Source: three-view drawing plus pictorial views. Frame: mm from the lowest corner of the part. A direction names the side the tool comes from. Give positions to 0.01 mm unless a question says otherwise; leave off trailing zeros. Loops run counter-clockwise (first coordinate to the right, second up) from the corner with the lowest first, then second, coordinate; pieces in that order, holes last. Notation, with made-up numbers: (68, -10.5) - (90, -10.5) arc R19 cw to (90, -1.5) - close; hole circle Ø7 at (-26, -5). An arc over 180 degrees is marked (long way). One line per item, written item: value.
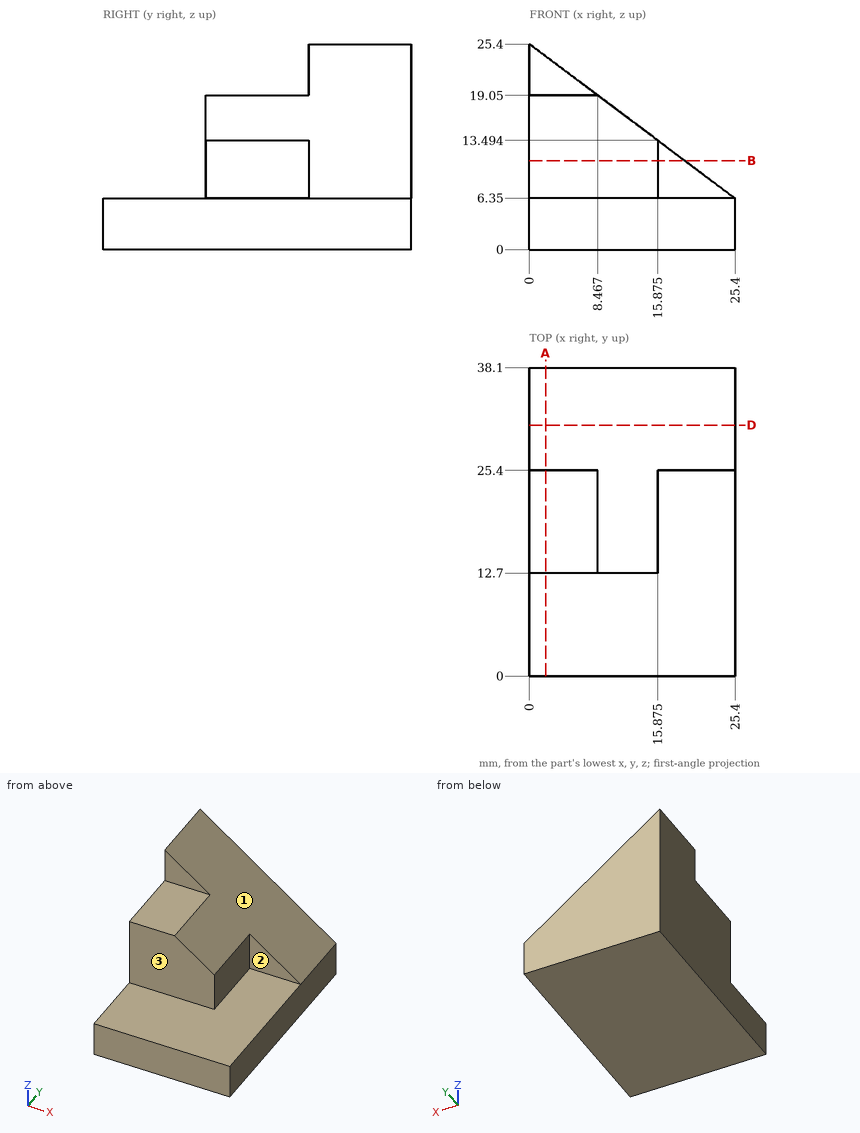
Item 1: Material intervals for L1, parallel to Z at x = 4.25, y = 6; L2, parallel to Z at x = 7.75, y = 14; L3, parallel to Y at x = 2.5, z = 10, sorted ascending.
Verdict:
L1: z = 0 to 6.35
L2: z = 0 to 19.05
L3: y = 12.7 to 38.1
Item 2: Section A-A, the plane x = 2. Output: boundary loops of the cut face in (y, z), and give its area (3 significant figures).
Verdict:
outline: (0, 0) - (38.1, 0) - (38.1, 23.9) - (25.4, 23.9) - (25.4, 19.05) - (12.7, 19.05) - (12.7, 6.35) - (0, 6.35) - close
area: 626 mm^2
Item 3: Section D-D, the plane y = 31. Output: boundary loops of the cut face in (x, z), and give its area (3 significant figures).
Verdict:
outline: (0, 0) - (25.4, 0) - (25.4, 6.35) - (0, 25.4) - close
area: 403 mm^2
Item 4: Access query for the marked faces 1, 2 and 3. Directions: +Z, -Z, +X, -X, +Y, -Y. A direction counts if a zero-diameter tool reaches every point of the face in a straight line with its end or side. Return the directions, or none.
Verdict:
face 1: +Z, +X, +Y, -Y
face 2: +Z, +X, -Y
face 3: +Z, +X, -X, -Y
Item 5: Section B-B, the plane z = 11. Output: boundary loops of the cut face in (x, y) (1 decimal).
Verdict:
outline: (0, 12.7) - (15.9, 12.7) - (15.9, 25.4) - (19.2, 25.4) - (19.2, 38.1) - (0, 38.1) - close
Item 6: Pin query (flat end, axial travel): P1, Ø7, axis at x = 5, y = 21, coming from the +Z side; P2, Ø2, axis at y = 17.5, z = 10.5, coming from the +X side (3 decimals); P3, Ø1.5, axis at x = 10.5, y = 8, coming from the +Z side. Return the tip coordinate at first contact, or that it passes through.
Verdict:
P1: stops at z = 19.05
P2: stops at x = 15.875
P3: stops at z = 6.35
